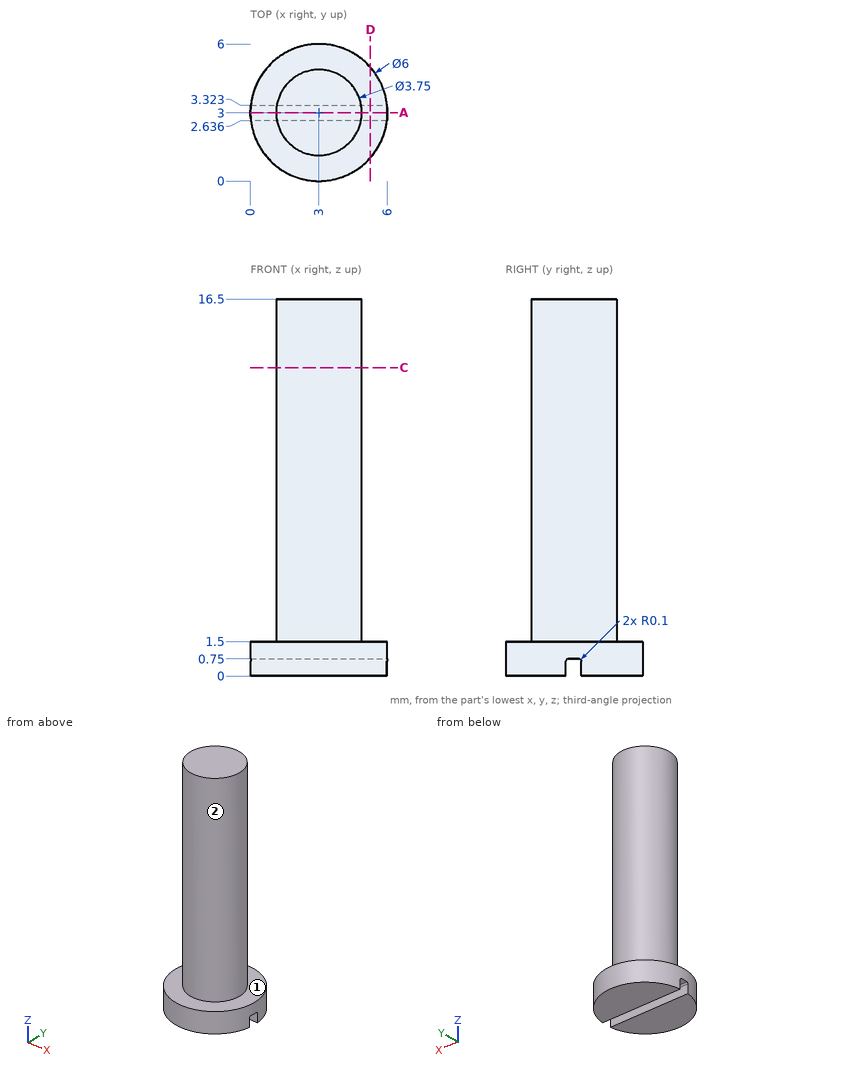
Print and shaded views of the part. All mm, measured from the part's lowest x, y and z. Coordinates: 2 decimals unless noted, no trailing zeros. Write each loop counter-clockwise with the first axis right and the second up, starting at its lowest first coordinate (ties: lowest second). Pieces come first, ordered by that corner, then holes. Notation, with made-up numbers: M 47.5,75.5 L 100.5,75.5 A29 cw 100.5,102.5 Z; hole C 32,76.5 d8. An arc over 180 degrees is marked long. Return JSON: item names as keys, results as strings.
1. Flat gauge pin, fed straight in: pin 1 Ø0.5 at (x, z) = (4.5, 0) entering from -Y. Where does the tip first touch, or does it go through?
Determined:
{"pin 1": "y = 0.27"}
2. Pull direction Y, two halves, no side cores. Call the marked faces 1 and 2: pulls with the +Y half, pulls with the -Y half, needs draft (parallel to the pull), parting line crosses it, or undercut.
Determined:
{"face 1": "needs draft", "face 2": "parting line crosses it"}
3. Saw through at D-D, the plane x = 5.25. Write the cut outline in (y, z).
Determined:
{"outline": "M 1.02,0 L 2.64,0 L 2.64,0.65 A0.1 cw 2.74,0.75 L 3.22,0.75 A0.1 cw 3.32,0.65 L 3.32,0 L 4.98,0 L 4.98,1.5 L 1.02,1.5 Z"}
4. Probe L1, parallel to Z at x = 4.5, y = 4.5; L2, parallel to Z at x = 1.5, y = 3.25; L3, parallel to Y at x = 2, z = 2.5. List the from-to ranges inside material, lowest first.
Determined:
{"L1": "0 to 1.5", "L2": "0.75 to 16.5", "L3": "1.41 to 4.59"}
5. Saw through at C-C, the plane z = 13.5. Write the cut outline in (x, y) (3 decimals), then the cut area to 3 significant figures.
Determined:
{"outline": "C 3,3 d3.75", "area": "11.0 mm²"}
6. Saw through at A-A, the plane y = 3. Write the cut outline in (x, z) (3 decimals).
Determined:
{"outline": "M 0,0.75 L 6,0.75 L 6,1.5 L 4.875,1.5 L 4.875,16.5 L 1.125,16.5 L 1.125,1.5 L 0,1.5 Z"}
